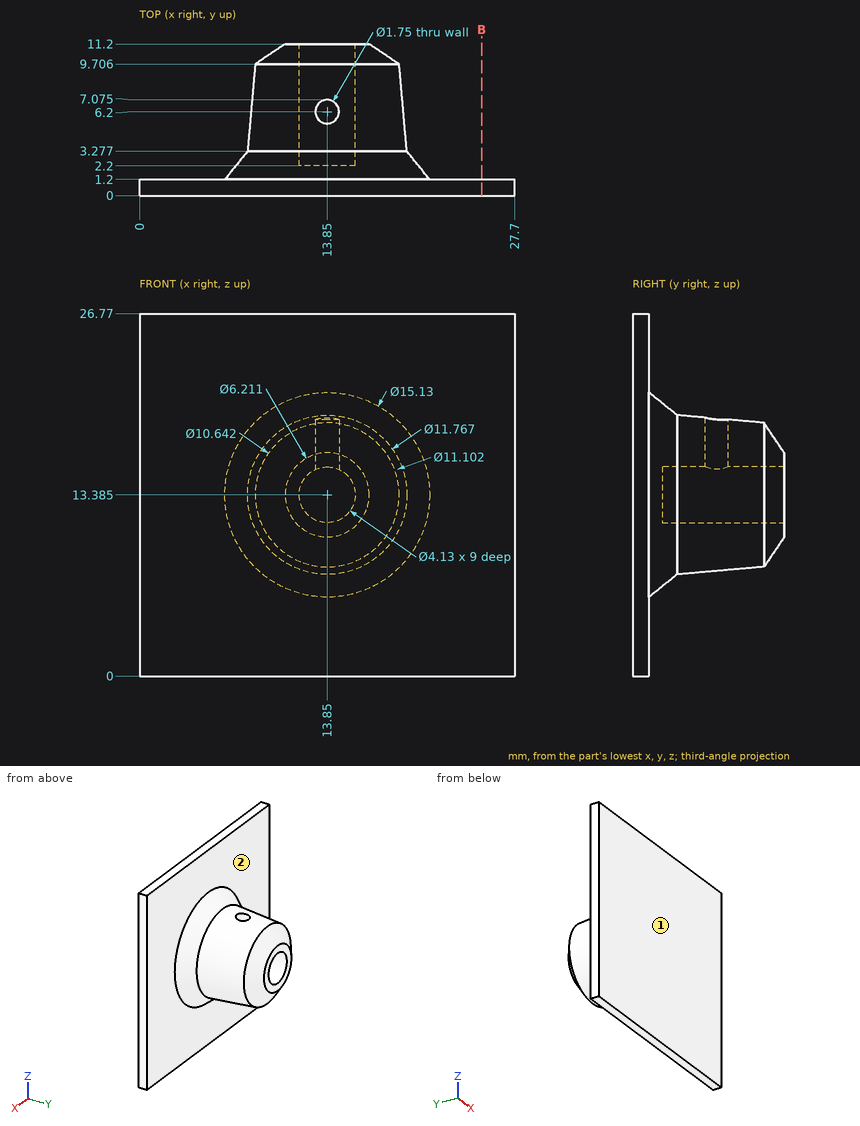
Drawing for the job (mm, zero at the part's lowest x, y, z). A direction names the side the tool comes from. Give positions to 0.01 mm unless a question says otherwise; leave off trailing zeros. Loops run counter-clockwise (first coordinate to the right, second up) from the corner with the lowest first, then second, coordinate; pieces in that order, holes last. Notation, with made-up numbers: M -10.75,52.5 L 28.25,52.5 A22 cw 28.25,84.5 Z; hole C 8.5,-24.75 d5. An arc over 180 degrees is marked long. One line per question, with ' | ' between items. Start each with the question number.
1. 3-axis set-ups, long thin cutter, end or side, ignore diameter. For the marked faces 1 and 2: which of +Z, -Z, +X, -X, +Y, -Y reach the whole face in a straight line?
2. Probe L1, parallel to X at y = 6.2, z = 17.8 (1 decimal); L2, parallel to Y at x = 19.25, z = 1; L3, parallel to X at y = 5.5, z = 15 (1 decimal). List the from-to ranges inside material, lowest first. Write a range as from..to.
3. Saw through at B-B on x = 25.25. Give the cut face in (y, z).
4. Flat gauge pins, fed straight in: pin 1 (3 mm diameter, centred on x = 7, y = 4.5, fed in from +Z); pin 2 (1 mm diameter, centred on x = 5.5, z = 13.5, fed in from +Y); pin 3 (1.5 mm diameter, centred on x = 12.5, y = 8.5, fed in from +Z). Where does each tip first touch, or does it go through?
Result sheet:
1) face 1: +Z, -Z, +X, -X, -Y | face 2: +Y
2) L1: x = 10.4..13, 14.7..17.3 | L2: y = 0..1.2 | L3: x = 8.4..12.6, 15.1..19.3
3) outline: M 0,0 L 1.2,0 L 1.2,26.77 L 0,26.77 Z
4) pin 1: stops at z = 15.58 | pin 2: stops at y = 1.2 | pin 3: stops at z = 18.8
